CAD build for the part. Positions are in the model's coordinates, mm. A direction names the side the tool comes from. Give positions to 0.01 mm unless a question says otherwise; leave off trailing zeros. Loops run counter-clockwise (first coordinate to the right, second up) from the corner with the lowest first, then second, coordinate; pieces in that order, holes last.
```python
from build123d import *

# Parameters (mm, degrees)
SKETCH_1_W      = 23.5
SKETCH_1_H      = 34
EXTRUDE_1_DEPTH = 113
SKETCH_2_R      = 1.8
EXTRUDE_2_DEPTH = 5
SKETCH_3_W      = 13
SKETCH_3_H      = 8
EXTRUDE_3_DEPTH = 8
FILLET_1_R      = 10
FILLET_2_R      = 2


with BuildPart() as part:
    # ｽｹｯﾁ1 → ﾎﾞｽ - 押し出し1 (new body)
    with BuildSketch(Plane(origin=(0, 0, 0), x_dir=(1, 0, 0), z_dir=(0, 1, 0))):
        Rectangle(SKETCH_1_W, SKETCH_1_H)
    extrude(amount=EXTRUDE_1_DEPTH)

    # ｽｹｯﾁ2 → ﾎﾞｽ - 押し出し2 (add)
    with BuildSketch(Plane.XY.offset(17)):
        with Locations(Location((-2, 103, 0), (0, 0, 180))):
            Circle(SKETCH_2_R)
        with Locations(Location((2, 103, 0), (0, 0, 180))):
            Circle(SKETCH_2_R)
    extrude(amount=EXTRUDE_2_DEPTH)

    # ｽｹｯﾁ3 → ﾎﾞｽ - 押し出し3 (add)
    with BuildSketch(Plane(origin=(0, 0, -17), x_dir=(-1, 0, 0), z_dir=(0, 0, -1))):
        with Locations((0, 107)):
            Rectangle(SKETCH_3_W, SKETCH_3_H)
    extrude(amount=EXTRUDE_3_DEPTH)

    # ﾌｨﾚｯﾄ1
    fillet_1_edges = [part.edges().sort_by_distance(p)[0] for p in [
        (-11.75, 113, 0),
        (11.75, 113, 0),
        (-11.75, 0, 0),
        (11.75, 0, 0),
    ]]
    fillet(fillet_1_edges, radius=FILLET_1_R)

    # ﾌｨﾚｯﾄ2
    # the kernel refuses this fillet: 2 mm, written as the material it takes off along each edge
    with BuildSketch(Plane(origin=(11.75, 10, -17), x_dir=(-1, 0, 0), z_dir=(0, 1, 0)), Plane(origin=(11.75, 10, 17), x_dir=(0, 0, -1), z_dir=(0, 1, 0))) as fillet_2_piece_1:
        with BuildLine():
            CenterArc((FILLET_2_R, FILLET_2_R), FILLET_2_R, 180, 90)
            Line((0, FILLET_2_R), (0, 0))
            Line((0, 0), (FILLET_2_R, 0))
        make_face()
    extrude(amount=93, mode=Mode.SUBTRACT)
    with BuildSketch(Plane(origin=(-1.75, 0, -17), x_dir=(0, 1, 0), z_dir=(1, 0, 0)), Plane(origin=(1.75, 113, 17), x_dir=(0, 0, -1), z_dir=(-1, 0, 0))) as fillet_2_piece_2:
        with BuildLine():
            CenterArc((FILLET_2_R, FILLET_2_R), FILLET_2_R, 180, 90)
            Line((0, FILLET_2_R), (0, 0))
            Line((0, 0), (FILLET_2_R, 0))
        make_face()
    extrude(amount=3.5, mode=Mode.SUBTRACT)
    with BuildSketch(Plane(origin=(-11.75, 10, -17), x_dir=(1, 0, 0), z_dir=(0, 1, 0)), Plane(origin=(-11.75, 10, 17), x_dir=(0, 0, -1), z_dir=(0, 1, 0))) as fillet_2_piece_3:
        with BuildLine():
            CenterArc((FILLET_2_R, -FILLET_2_R), FILLET_2_R, 90, 90)
            Line((0, -FILLET_2_R), (0, 0))
            Line((0, 0), (FILLET_2_R, 0))
        make_face()
    extrude(amount=93, mode=Mode.SUBTRACT)
    with BuildSketch(Plane(origin=(-1.75, 113, -17), x_dir=(0, -1, 0), z_dir=(1, 0, 0)), Plane(origin=(1.75, 0, 17), x_dir=(0, 0, -1), z_dir=(-1, 0, 0))) as fillet_2_piece_4:
        with BuildLine():
            CenterArc((FILLET_2_R, -FILLET_2_R), FILLET_2_R, 90, 90)
            Line((0, -FILLET_2_R), (0, 0))
            Line((0, 0), (FILLET_2_R, 0))
        make_face()
    extrude(amount=3.5, mode=Mode.SUBTRACT)
    with BuildSketch(Plane(origin=(1.75, 103, -17), x_dir=(0, 1, 0), z_dir=(-1, 0, 0))) as fillet_2_piece_5_section:
        with BuildLine():
            CenterArc((10 - FILLET_2_R, -FILLET_2_R), FILLET_2_R, 0, 90)
            Line((10, -FILLET_2_R), (10, 0))
            Line((10, 0), (10 - FILLET_2_R, 0))
        make_face()
    fillet_2_piece_5 = revolve(axis=Axis((1.75, 103, -17), (0, 0, -1)), revolution_arc=90, mode=Mode.PRIVATE)
    fillet_2_piece_5 = split(fillet_2_piece_5, bisect_by=Plane(origin=(4.101759822, 111, -16.527412799), z_dir=(0, 1, 0)), keep=Keep.TOP, mode=Mode.PRIVATE)
    fillet_2_piece_5 = split(fillet_2_piece_5, bisect_by=Plane(origin=(6.5, 112.1945957, -16.527412799), z_dir=(-1, 0, 0)), keep=Keep.TOP, mode=Mode.PRIVATE)
    add(fillet_2_piece_5, mode=Mode.SUBTRACT)
    with BuildSketch(Plane(origin=(1.75, 103, -17), x_dir=(0, 1, 0), z_dir=(-1, 0, 0))) as fillet_2_piece_6_section:
        with BuildLine():
            CenterArc((10 - FILLET_2_R, -FILLET_2_R), FILLET_2_R, 0, 90)
            Line((10, -FILLET_2_R), (10, 0))
            Line((10, 0), (10 - FILLET_2_R, 0))
        make_face()
    fillet_2_piece_6 = revolve(axis=Axis((1.75, 103, -17), (0, 0, -1)), revolution_arc=90, mode=Mode.PRIVATE)
    fillet_2_piece_6 = split(fillet_2_piece_6, bisect_by=Plane(origin=(9.944543227, 111, -16.429177526), z_dir=(0, -1, 0)), keep=Keep.TOP, mode=Mode.PRIVATE)
    fillet_2_piece_6 = split(fillet_2_piece_6, bisect_by=Plane(origin=(6.5, 107.664638262, -16.429177526), z_dir=(1, 0, 0)), keep=Keep.TOP, mode=Mode.PRIVATE)
    add(fillet_2_piece_6, mode=Mode.SUBTRACT)
    with BuildSketch(Plane(origin=(1.75, 103, -17), x_dir=(0, 1, 0), z_dir=(-1, 0, 0))) as fillet_2_piece_7_section:
        with BuildLine():
            CenterArc((10 - FILLET_2_R, -FILLET_2_R), FILLET_2_R, 0, 90)
            Line((10, -FILLET_2_R), (10, 0))
            Line((10, 0), (10 - FILLET_2_R, 0))
        make_face()
    fillet_2_piece_7 = revolve(axis=Axis((1.75, 103, -17), (0, 0, -1)), revolution_arc=90, mode=Mode.PRIVATE)
    fillet_2_piece_7 = split(fillet_2_piece_7, bisect_by=Plane(origin=(6.999362203, 111, -16.337935444), z_dir=(0, 1, 0)), keep=Keep.TOP, mode=Mode.PRIVATE)
    fillet_2_piece_7 = split(fillet_2_piece_7, bisect_by=Plane(origin=(6.5, 111.322531281, -16.337935444), z_dir=(1, 0, 0)), keep=Keep.TOP, mode=Mode.PRIVATE)
    add(fillet_2_piece_7, mode=Mode.SUBTRACT)
    with BuildSketch(Plane(origin=(-1.75, 103, -17), x_dir=(-1, 0, 0), z_dir=(0, -1, 0))) as fillet_2_piece_8_section:
        with BuildLine():
            CenterArc((10 - FILLET_2_R, -FILLET_2_R), FILLET_2_R, 0, 90)
            Line((10, -FILLET_2_R), (10, 0))
            Line((10, 0), (10 - FILLET_2_R, 0))
        make_face()
    fillet_2_piece_8 = revolve(axis=Axis((-1.75, 103, -17), (0, 0, -1)), revolution_arc=90, mode=Mode.PRIVATE)
    fillet_2_piece_8 = split(fillet_2_piece_8, bisect_by=Plane(origin=(-6.5, 107.664638263, -16.429177529), z_dir=(-1, 0, 0)), keep=Keep.TOP, mode=Mode.PRIVATE)
    fillet_2_piece_8 = split(fillet_2_piece_8, bisect_by=Plane(origin=(-9.94454323, 111, -16.429177529), z_dir=(0, -1, 0)), keep=Keep.TOP, mode=Mode.PRIVATE)
    add(fillet_2_piece_8, mode=Mode.SUBTRACT)
    with BuildSketch(Plane(origin=(-1.75, 103, -17), x_dir=(-1, 0, 0), z_dir=(0, -1, 0))) as fillet_2_piece_9_section:
        with BuildLine():
            CenterArc((10 - FILLET_2_R, -FILLET_2_R), FILLET_2_R, 0, 90)
            Line((10, -FILLET_2_R), (10, 0))
            Line((10, 0), (10 - FILLET_2_R, 0))
        make_face()
    fillet_2_piece_9 = revolve(axis=Axis((-1.75, 103, -17), (0, 0, -1)), revolution_arc=90, mode=Mode.PRIVATE)
    fillet_2_piece_9 = split(fillet_2_piece_9, bisect_by=Plane(origin=(-6.5, 111.32253137, -16.337935534), z_dir=(-1, 0, 0)), keep=Keep.TOP, mode=Mode.PRIVATE)
    fillet_2_piece_9 = split(fillet_2_piece_9, bisect_by=Plane(origin=(-6.999362106, 111, -16.337935534), z_dir=(0, 1, 0)), keep=Keep.TOP, mode=Mode.PRIVATE)
    add(fillet_2_piece_9, mode=Mode.SUBTRACT)
    with BuildSketch(Plane(origin=(-1.75, 103, -17), x_dir=(-1, 0, 0), z_dir=(0, -1, 0))) as fillet_2_piece_10_section:
        with BuildLine():
            CenterArc((10 - FILLET_2_R, -FILLET_2_R), FILLET_2_R, 0, 90)
            Line((10, -FILLET_2_R), (10, 0))
            Line((10, 0), (10 - FILLET_2_R, 0))
        make_face()
    fillet_2_piece_10 = revolve(axis=Axis((-1.75, 103, -17), (0, 0, -1)), revolution_arc=90, mode=Mode.PRIVATE)
    fillet_2_piece_10 = split(fillet_2_piece_10, bisect_by=Plane(origin=(-6.5, 112.194595792, -16.527412821), z_dir=(1, 0, 0)), keep=Keep.TOP, mode=Mode.PRIVATE)
    fillet_2_piece_10 = split(fillet_2_piece_10, bisect_by=Plane(origin=(-4.101760011, 111, -16.527412821), z_dir=(0, 1, 0)), keep=Keep.TOP, mode=Mode.PRIVATE)
    add(fillet_2_piece_10, mode=Mode.SUBTRACT)
    with BuildSketch(Plane(origin=(-1.75, 10, -17), x_dir=(-1, 0, 0), z_dir=(0, 1, 0))) as fillet_2_piece_11:
        with BuildLine():
            CenterArc((10 - FILLET_2_R, FILLET_2_R), FILLET_2_R, 270, 90)
            Line((10, FILLET_2_R), (10, 0))
            Line((10, 0), (10 - FILLET_2_R, 0))
        make_face()
    revolve(axis=Axis((-1.75, 10, -17), (0, 0, 1)), revolution_arc=90, mode=Mode.SUBTRACT)
    with BuildSketch(Plane(origin=(1.75, 10, -17), x_dir=(0, -1, 0), z_dir=(-1, 0, 0))) as fillet_2_piece_12:
        with BuildLine():
            CenterArc((10 - FILLET_2_R, FILLET_2_R), FILLET_2_R, 270, 90)
            Line((10, FILLET_2_R), (10, 0))
            Line((10, 0), (10 - FILLET_2_R, 0))
        make_face()
    revolve(axis=Axis((1.75, 10, -17), (0, 0, 1)), revolution_arc=90, mode=Mode.SUBTRACT)
    with BuildSketch(Plane(origin=(1.75, 103, 17), x_dir=(0, 1, 0), z_dir=(-1, 0, 0))) as fillet_2_piece_13:
        with BuildLine():
            CenterArc((10 - FILLET_2_R, FILLET_2_R), FILLET_2_R, 270, 90)
            Line((10 - FILLET_2_R, 0), (10, 0))
            Line((10, 0), (10, FILLET_2_R))
        make_face()
    revolve(axis=Axis((1.75, 103, 17), (0, 0, -1)), revolution_arc=90, mode=Mode.SUBTRACT)
    with BuildSketch(Plane(origin=(-1.75, 103, 17), x_dir=(-1, 0, 0), z_dir=(0, -1, 0))) as fillet_2_piece_14:
        with BuildLine():
            CenterArc((10 - FILLET_2_R, FILLET_2_R), FILLET_2_R, 270, 90)
            Line((10 - FILLET_2_R, 0), (10, 0))
            Line((10, 0), (10, FILLET_2_R))
        make_face()
    revolve(axis=Axis((-1.75, 103, 17), (0, 0, -1)), revolution_arc=90, mode=Mode.SUBTRACT)
    with BuildSketch(Plane(origin=(-1.75, 10, 17), x_dir=(-1, 0, 0), z_dir=(0, 1, 0))) as fillet_2_piece_15:
        with BuildLine():
            CenterArc((10 - FILLET_2_R, -FILLET_2_R), FILLET_2_R, 0, 90)
            Line((10 - FILLET_2_R, 0), (10, 0))
            Line((10, 0), (10, -FILLET_2_R))
        make_face()
    revolve(axis=Axis((-1.75, 10, 17), (0, 0, 1)), revolution_arc=90, mode=Mode.SUBTRACT)
    with BuildSketch(Plane(origin=(1.75, 10, 17), x_dir=(0, -1, 0), z_dir=(-1, 0, 0))) as fillet_2_piece_16:
        with BuildLine():
            CenterArc((10 - FILLET_2_R, -FILLET_2_R), FILLET_2_R, 0, 90)
            Line((10 - FILLET_2_R, 0), (10, 0))
            Line((10, 0), (10, -FILLET_2_R))
        make_face()
    revolve(axis=Axis((1.75, 10, 17), (0, 0, 1)), revolution_arc=90, mode=Mode.SUBTRACT)


solid = part.part
```
1. Saw through at B-B, the plane y = 26. List the corners of the cut face in (x, z), and give its area (3 significant figures).
Responses:
outline: (-11.75, -15) arc R2 ccw to (-9.75, -17) - (9.75, -17) arc R2 ccw to (11.75, -15) - (11.75, 15) arc R2 ccw to (9.75, 17) - (-9.75, 17) arc R2 ccw to (-11.75, 15) - close
area: 796 mm2
2. Probe line 1 along Z through (x, y) = (9.5, 48); line 2 along Y through (x, z) = (-2, -14); line 3 along Y through (x, z) = (-2.75, -23). List the from-to ranges inside material, lowest first.
Responses:
line 1: z = -17 to 17
line 2: y = 0 to 113
line 3: y = 103 to 111
3. Drop flat-ended pins along their axis: pin 1 (8 mm diameter, centred on x = 0, y = 74, fed in from +Z); pin 2 (2.5 mm diameter, centred on x = -2, z = -22, fed in from +Y); pin 3 (6.5 mm diameter, centred on y = 106, z = -20, fed in from -X). Give the stop position or say it passes through.
Responses:
pin 1: stops at z = 17
pin 2: stops at y = 111
pin 3: stops at x = -10.29
4. Saw through at C-C, the plane z = -21.5. List the corners of the cut face in (x, y).
Responses:
outline: (-6.5, 103) - (6.5, 103) - (6.5, 111) - (-6.5, 111) - close
5. Saw through at A-A, the plane z = 18. List the corners of the cut face in (x, y), and give its area (3 significant figures).
Responses:
outline: circle Ø3.6 at (-2, 103); circle Ø3.6 at (2, 103)
area: 20.4 mm2
6. Tool access for faces 5 (the face through (-8.9, 109.99, -0.21)), 6 (the face through (1.169, 104.597, 19.465)): list every direction of +Z, -Z, +X, -X, +Y, -Y with a clear straight run to the whole face (end or side of a thin tool).
Responses:
face 5: +Z, -Z, -X, +Y
face 6: +Z
7. Pull direction X, two halves, no side cores. Call faces 1 (the face through (8.74, 110.15, -0.21)), 2 (the face through (-11.18, 55.85, 16.4)), 3 (the face through (-2.831, 104.597, 19.465)), 4 (the face through (0, 0, 0)): released by +X, released by -X, zero draft, split by the parting line, or undercut.
Responses:
face 1: released by +X
face 2: released by -X
face 3: undercut
face 4: zero draft
